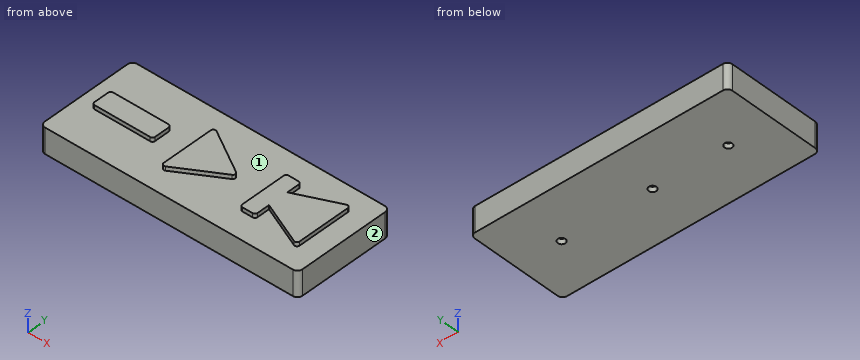
from build123d import *

# Parameters (mm, degrees)
BOSS_EXTRUDE1_DEPTH = 5
SKETCH6_R           = 0.75
CUT_EXTRUDE1_DEPTH  = 1
BOSS_EXTRUDE3_DEPTH = 0.8


with BuildPart() as part:
    # Sketch3 → Boss-Extrude1 (new body)
    with BuildSketch(Plane.XY):
        with BuildLine():
            Line((-24, 10), (25, 10))
            ThreePointArc((25, 10), (25.707106781, 9.707106781), (26, 9))
            Line((26, 9), (26, -9))
            ThreePointArc((26, -9), (25.707106781, -9.707106781), (25, -10))
            Line((25, -10), (-24, -10))
            ThreePointArc((-24, -10), (-24.707106781, -9.707106781), (-25, -9))
            Line((-25, -9), (-25, 9))
            ThreePointArc((-25, 9), (-24.707106781, 9.707106781), (-24, 10))
        make_face()
    extrude(amount=BOSS_EXTRUDE1_DEPTH)

    # Sketch6 → Cut-Extrude1 (cut)
    with BuildSketch(Plane.XY):
        with Locations((-16, 0)):
            Circle(SKETCH6_R)
        with Locations((-1, 0)):
            Circle(SKETCH6_R)
        with Locations((17, 0)):
            Circle(SKETCH6_R)
    extrude(amount=CUT_EXTRUDE1_DEPTH, mode=Mode.SUBTRACT)

    # Sketch4 → Boss-Extrude3 (add)
    with BuildSketch(Plane.XY.offset(5)):
        with BuildLine():
            Line((-5, 5.116904811), (-5, -5.116904811))
            ThreePointArc((-5, -5.116904811), (-4.746349407, -5.552004764), (-4.242752122, -5.545651273))
            Line((-4.242752122, -5.545651273), (4.285422562, -0.428746463))
            ThreePointArc((4.285422562, -0.428746463), (4.528174684, 0), (4.285422562, 0.428746463))
            Line((4.285422562, 0.428746463), (-4.242752122, 5.545651273))
            ThreePointArc((-4.242752122, 5.545651273), (-4.746349407, 5.552004764), (-5, 5.116904811))
        make_face()
        with BuildLine():
            Line((10, 4.5), (10, -4.5))
            ThreePointArc((10, -4.5), (10.146446609, -4.853553391), (10.5, -5))
            Line((10.5, -5), (12.5, -5))
            ThreePointArc((12.5, -5), (12.853553391, -4.853553391), (13, -4.5))
            Line((13, -4.5), (13, -2))
            Line((13, -2), (21.296930767, -5.687524785))
            ThreePointArc((21.296930767, -5.687524785), (21.77245677, -5.64986513), (22, -5.230619011))
            Line((22, -5.230619011), (22, 5.230619011))
            ThreePointArc((22, 5.230619011), (21.77245677, 5.64986513), (21.296930767, 5.687524785))
            Line((21.296930767, 5.687524785), (13, 2))
            Line((13, 2), (13, 4.5))
            ThreePointArc((13, 4.5), (12.853553391, 4.853553391), (12.5, 5))
            Line((12.5, 5), (10.5, 5))
            ThreePointArc((10.5, 5), (10.146446609, 4.853553391), (10, 4.5))
        make_face()
        with BuildLine():
            Line((-21.5, 2), (-10.5, 2))
            ThreePointArc((-10.5, 2), (-10.146446609, 1.853553391), (-10, 1.5))
            Line((-10, 1.5), (-10, -1.5))
            ThreePointArc((-10, -1.5), (-10.146446609, -1.853553391), (-10.5, -2))
            Line((-10.5, -2), (-21.5, -2))
            ThreePointArc((-21.5, -2), (-21.853553391, -1.853553391), (-22, -1.5))
            Line((-22, -1.5), (-22, 1.5))
            ThreePointArc((-22, 1.5), (-21.853553391, 1.853553391), (-21.5, 2))
        make_face()
    extrude(amount=BOSS_EXTRUDE3_DEPTH)


solid = part.part
Source: CAD feature listing. Evaluate the final solid. Frame: model axes, mm. Face numbers are marked on the shaded views. A direction names the side the tool comes from. Give positions to 0.01 mm unless a question says otherwise; leave off trailing zeros. Order: outer loops, then holes, each group sorted by start corner. A loop starts at its lowest first (then second) coordinate and runs counter-clockwise, first axis right, second up. Notation, with made-up numbers: (-9.75, 43.25) -> (39.25, 43.25) arc R14 ccw to (39.25, 66.25) -> close; hole circle Ø1 at (-38.75, 85). An arc over 180 degrees is marked (long way). Write item = value, one per line.
Item 1: Contact query for flat-ended pins moving along their axis: pin 1 (0.8 mm diameter, centred on x = -1, y = 0, fed in from -Z); pin 2 (2 mm diameter, centred on x = -15.5, y = -7.5, fed in from -Z); pin 3 (3 mm diameter, centred on x = -16, y = 7, fed in from +Z); pin 4 (0.9 mm diameter, centred on x = -14.5, z = 5.5, fed in from -Y). Output: stop coordinate, or through.
Check result:
pin_1 = 1
pin_2 = 0
pin_3 = 5
pin_4 = -2
Item 2: Section query B-B (x = -18.5). Output: boundary loops of the cut face in (y, z), then the cut area to 3 significant figures.
Check result:
outline = (-10, 0) -> (10, 0) -> (10, 5) -> (2, 5) -> (2, 5.8) -> (-2, 5.8) -> (-2, 5) -> (-10, 5) -> close
area = 103 mm²
Item 3: Ray query, probe 1 along Y at (x, z) = (-1, 0.45); probe 2 along Z at (x, y) = (-17, -7.5). Return the intervals inside material, ascending.
Check result:
probe_1 = -10 to -0.75, 0.75 to 10
probe_2 = 0 to 5
Item 4: Section query D-D (x = 18.5). Output: boundary loops of the cut face in (y, z), then the cut area to 3 significant figures.
Check result:
outline = (-10, 0) -> (10, 0) -> (10, 5) -> (4.44, 5) -> (4.44, 5.8) -> (-4.44, 5.8) -> (-4.44, 5) -> (-10, 5) -> close
area = 107 mm²
Item 5: Section query C-C (y = 3.75). Output: boundary loops of the cut face in (x, z), then the cut area to 3 significant figures.
Check result:
outline = (-25, 0) -> (26, 0) -> (26, 5) -> (22, 5) -> (22, 5.8) -> (16.94, 5.8) -> (16.94, 5) -> (13, 5) -> (13, 5.8) -> (10, 5.8) -> (10, 5) -> (-1.25, 5) -> (-1.25, 5.8) -> (-5, 5.8) -> (-5, 5) -> (-25, 5) -> close
area = 264 mm²
Item 6: Section query A-A (y = -3). Output: boundary loops of the cut face in (x, z).
Check result:
outline = (-25, 0) -> (26, 0) -> (26, 5) -> (22, 5) -> (22, 5.8) -> (15.25, 5.8) -> (15.25, 5) -> (13, 5) -> (13, 5.8) -> (10, 5.8) -> (10, 5) -> (0, 5) -> (0, 5.8) -> (-5, 5.8) -> (-5, 5) -> (-25, 5) -> close
Item 7: Set-up query: the marked faces 1 and 2. Return all of +Z, -Z, +X, -X, +Y, -Y with unobstructed straight access to the full face (end or side cutting, diameter ignored); none if empty.
Check result:
face_1 = +Z
face_2 = +Z, -Z, +X, +Y, -Y
